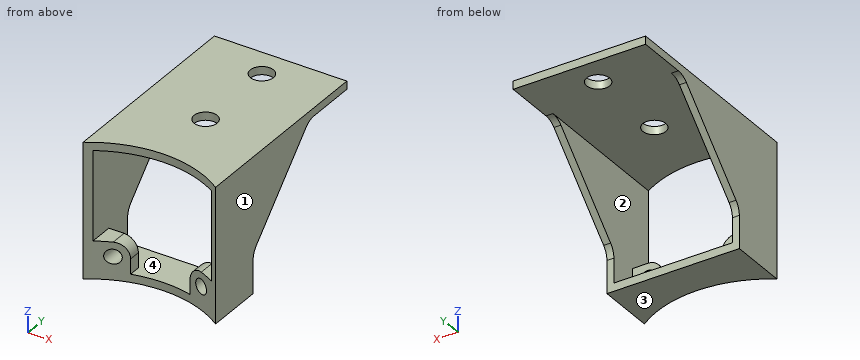
```python
from build123d import *

# Parameters (mm, degrees)
SKETCH_1_W          = 22.9
SKETCH_1_H          = 23.3
SKETCH_1_W_2        = 20.5
SKETCH_1_H_2        = 20.5
EXTRUDE_1_DEPTH     = 10
SKETCH_1_4_R        = 1.27
EXTRUDE_2_DEPTH     = 5
EXTRUDE_3_DEPTH     = 10
SKETCH_3_W          = 22.9
SKETCH_3_H          = 1.4
EXTRUDE_4_DEPTH     = 25
CUT_EXTRUDE_1_REACH = 25.3
SKETCH_4_R          = 20
SKETCH_5_R          = 2
CUT_EXTRUDE_2_DEPTH = 2.4000001
CHAMFER_1_SIZE      = 15
FILLET_1_R          = 3


with BuildPart() as part:
    # Sketch 1 → Extrude 1 (new body)
    with BuildSketch(Plane(origin=(0, 0, 0), x_dir=(1, 0, 0), z_dir=(0, 1, 0))):
        Rectangle(SKETCH_1_W, SKETCH_1_H)
        Rectangle(SKETCH_1_W_2, SKETCH_1_H_2, mode=Mode.SUBTRACT)
        Polygon((10.25, -10.25), (-10.25, -10.25), (-11.45, -10.25), (-11.45, -11.65), (11.45, -11.65), (11.45, -10.25), align=None)
    extrude(amount=EXTRUDE_1_DEPTH)

    # Sketch 1_4 → Extrude 2 (add)
    with BuildSketch(Plane(origin=(0, 0, 0), x_dir=(1, 0, 0), z_dir=(0, 1, 0))):
        with BuildLine():
            Line((-5.15, 10.25), (-10.25, 10.25))
            Line((-10.25, 10.25), (-10.25, 5.18))
            Line((-10.25, 5.18), (-7.62, 5.18))
            ThreePointArc((-7.62, 5.18), (-5.87344625, 5.90344625), (-5.15, 7.65))
            Line((-5.15, 7.65), (-5.15, 10.25))
        make_face()
        with Locations((-7.62, 7.65)):
            Circle(SKETCH_1_4_R, mode=Mode.SUBTRACT)
        with BuildLine():
            Line((10.25, 10.25), (5.15, 10.25))
            Line((5.15, 10.25), (5.15, 7.65))
            ThreePointArc((5.15, 7.65), (5.87344625, 5.90344625), (7.62, 5.18))
            Line((7.62, 5.18), (10.25, 5.18))
            Line((10.25, 5.18), (10.25, 10.25))
        make_face()
        with Locations((7.62, 7.65)):
            Circle(SKETCH_1_4_R, mode=Mode.SUBTRACT)
    extrude(amount=EXTRUDE_2_DEPTH)

    # Sketch 1_5 → Extrude 3 (add)
    with BuildSketch(Plane(origin=(0, 0, 0), x_dir=(1, 0, 0), z_dir=(0, 1, 0))):
        Polygon((10.25, -10.25), (-10.25, -10.25), (-11.45, -10.25), (-11.45, -11.65), (11.45, -11.65), (11.45, -10.25), align=None)
    extrude(amount=EXTRUDE_3_DEPTH)

    # Sketch 3 → Extrude 4 (add)
    with BuildSketch(Plane(origin=(0, 10, 0), x_dir=(1, 0, 0), z_dir=(0, 1, 0))):
        with Locations((0, -10.95)):
            Rectangle(SKETCH_3_W, SKETCH_3_H)
    extrude(amount=EXTRUDE_4_DEPTH)

    # Sketch 4 → Cut-Extrude 1 (cut, up to next)
    with BuildSketch(Plane(origin=(0, 0, -11.65), x_dir=(-1, 0, 0), z_dir=(0, 0, -1)), mode=Mode.PRIVATE) as cut_extrude_1_sk1:
        with Locations((0, -16.398094401)):
            Circle(SKETCH_4_R)
    cut_extrude_1_tool1 = extrude(cut_extrude_1_sk1.sketch, amount=-CUT_EXTRUDE_1_REACH, mode=Mode.PRIVATE) & part.part
    add(cut_extrude_1_tool1.solids().sort_by_distance((0, -16.398094, -11.65))[0], mode=Mode.SUBTRACT)

    # Sketch 5 → Cut-Extrude 2 (cut, through all)
    with BuildSketch(Plane(origin=(0, 0, 10.25), x_dir=(-1, 0, 0), z_dir=(0, 0, -1))):
        with Locations((0, 15)):
            Circle(SKETCH_5_R)
        with Locations((0, 30)):
            Circle(SKETCH_5_R)
    extrude(amount=-CUT_EXTRUDE_2_DEPTH, mode=Mode.SUBTRACT)

    # Chamfer 1
    chamfer_1_edges = [part.edges().sort_by_distance(p)[0] for p in [
        (-10.85, 10, 10.25),
        (10.85, 10, 10.25),
    ]]
    chamfer(chamfer_1_edges, length=CHAMFER_1_SIZE)

    # Fillet 1
    fillet_1_edges = [part.edges().sort_by_distance(p)[0] for p in [
        (-10.85, 25, 10.25),
        (10.85, 25, 10.25),
        (-10.85, 10, -4.75),
        (10.85, 10, -4.75),
    ]]
    fillet(fillet_1_edges, radius=FILLET_1_R)


solid = part.part
```
The listing builds one solid part. Answer for the finished solid, in the listing's coordinates (mm). Face numbers are marked on the shaded views. Coordinates: 2 decimals unless noted, no trailing zeros. Write each loop counter-clockwise with the first axis right and the second up, starting at its lowest first coordinate (ties: lowest second). Pieces come first, ordered by that corner, then holes.
Q1. Section B-B, the plane z = 4.5 is taken. Write down the section's boundary in (x, y), then the cut area to 3 significant figures.
Returned:
outline: (-11.45, 0) arc R20 cw to (-10.25, 0.78) - (-10.25, 19.25) - (-11.45, 19.25) - close; (10.25, 0.78) arc R20 cw to (11.45, 0) - (11.45, 19.25) - (10.25, 19.25) - close
area: 45.2 mm2
Q2. Find the intervals of material crossed by line 1 along Z through (x, y) = (-7.62, 3.55); line 2 along Y through (x, z) = (0, 11); line 3 along Z through (x, y) = (-9.25, 5.5), in increasing order.
Returned:
line 1: z = -11.65 to -8.92, -6.38 to -5.18, 10.25 to 11.65
line 2: y = 3.6 to 13, 17 to 28, 32 to 35
line 3: z = -11.65 to -10.25, 10.25 to 11.65
Q3. The mould has two halves that part along X. Classify the marked faces 1, 2, 3 and 4: released by +X, released by -X, zero draft, split by the parting line, or undercut.
Returned:
face 1: released by +X
face 2: undercut
face 3: zero draft
face 4: undercut
Q4. Section A-A, the plane y = 30 is taken. Write down the section's boundary in (x, z), then the cut area to 3 significant figures.
Returned:
outline: (-11.45, 10.25) - (-2, 10.25) - (-2, 11.65) - (-11.45, 11.65) - close; (2, 10.25) - (11.45, 10.25) - (11.45, 11.65) - (2, 11.65) - close
area: 26.5 mm2
Q5. Section D-D, the plane z = -7.25 is taken. Write down the section's boundary in (x, y).
Returned:
outline: (-11.45, 0) arc R20 cw to (-8.83, 1.55) - (-8.83, 5) - (-10.25, 5) - (-10.25, 10) - (-11.45, 10) - close; (-6.41, 2.55) arc R20 cw to (-5.18, 2.92) - (-5.18, 5) - (-6.41, 5) - close; (5.18, 2.92) arc R20 cw to (6.41, 2.55) - (6.41, 5) - (5.18, 5) - close; (8.83, 1.55) arc R20 cw to (11.45, 0) - (11.45, 10) - (10.25, 10) - (10.25, 5) - (8.83, 5) - close
Q6. Section C-C, the plane x = 1 is taken. Write down the section's boundary in (y, z), then the cut area to 3 significant figures.
Returned:
outline: (3.58, -11.65) - (10, -11.65) - (10, -10.25) - (3.58, -10.25) - close; (3.58, 10.25) - (13.27, 10.25) - (13.27, 11.65) - (3.58, 11.65) - close; (16.73, 10.25) - (28.27, 10.25) - (28.27, 11.65) - (16.73, 11.65) - close; (31.73, 10.25) - (35, 10.25) - (35, 11.65) - (31.73, 11.65) - close
area: 43.3 mm2
Q7. Given P1, Ø12, axis at x = -0.5, z = 2.5, coming from the +Y side; P2, Ø4, axis at x = 7, z = -7, coming from the +Y side; P3, Ø4, axis at x = -7.62, z = -7.65, coming from the -Y side, each flat-ended and moving along its own axis, determine where each tip first touches the part or whether it passes through.
Returned:
P1: passes through
P2: stops at y = 5
P3: stops at y = 1.14
